from build123d import *

# Parameters (mm, degrees)
SKETCH1_W           = 40
SKETCH1_H           = 28
BOSS_EXTRUDE1_DEPTH = 10
SKETCH2_W           = 40
SKETCH2_H           = 1.6
CUT_EXTRUDE1_DEPTH  = 5
SKETCH3_W           = 24
SKETCH3_H           = 10
CUT_EXTRUDE2_DEPTH  = 27.381811917
SKETCH4_W           = 4
SKETCH4_H           = 26.4
CUT_EXTRUDE3_DEPTH  = 5
FILLET1_R           = 2
FILLET2_R           = 1
CHAMFER2_SIZE       = 0.6


with BuildPart() as part:
    # Sketch1 → Boss-Extrude1 (new body)
    with BuildSketch(Plane(origin=(0, 0, 0), x_dir=(1, 0, 0), z_dir=(0, 1, 0))):
        Rectangle(SKETCH1_W, SKETCH1_H)
    extrude(amount=BOSS_EXTRUDE1_DEPTH)

    # Sketch2 → Cut-Extrude1 (cut)
    with BuildSketch(Plane.XZ):
        with Locations((0, 13.2)):
            Rectangle(SKETCH2_W, SKETCH2_H)
    extrude(amount=-CUT_EXTRUDE1_DEPTH, mode=Mode.SUBTRACT)

    # Sketch3 → Cut-Extrude2 (cut, through all)
    with BuildSketch(Plane(origin=(0, 10, 0), x_dir=(1, 0, 0), z_dir=(0, 1, 0))):
        with Locations((0, -14)):
            Rectangle(SKETCH3_W, SKETCH3_H)
    extrude(amount=-CUT_EXTRUDE2_DEPTH, mode=Mode.SUBTRACT)

    # Sketch4 → Cut-Extrude3 (cut)
    with BuildSketch(Plane.XZ):
        with Locations((-18, -0.8)):
            Rectangle(SKETCH4_W, SKETCH4_H)
        with Locations((18, -0.8)):
            Rectangle(SKETCH4_W, SKETCH4_H)
    extrude(amount=-CUT_EXTRUDE3_DEPTH, mode=Mode.SUBTRACT)

    # Fillet1
    fillet1_edges = [part.edges().sort_by_distance(p)[0] for p in [
        (12, 5, 9),
        (-12, 5, 9),
    ]]
    fillet(fillet1_edges, radius=FILLET1_R)

    # Fillet2
    fillet2_edges = [part.edges().sort_by_distance(p)[0] for p in [
        (12, 7.5, 14),
        (12, 2.5, 12.4),
        (-12, 7.5, 14),
        (-12, 2.5, 12.4),
        (-16, 2.5, 12.4),
        (-16, 2.5, -14),
        (16, 2.5, -14),
        (16, 2.5, 12.4),
        (20, 7.5, 14),
        (-20, 7.5, 14),
        (-20, 7.5, -14),
        (20, 7.5, -14),
    ]]
    fillet(fillet2_edges, radius=FILLET2_R)

    # Chamfer2
    chamfer2_edges = [part.edges().sort_by_distance(p)[0] for p in [
        (0, 0, -14),
        (0, 10, -14),
        (17, 5, -14),
        (-12, 10, 12),
        (12, 10, 12),
        (16, 10, 14),
        (20, 10, 0),
        (-16, 10, 14),
        (-12.292893219, 10, 13.707106781),
        (-19.707106781, 10, 13.707106781),
        (12.292893219, 10, 13.707106781),
        (19.707106781, 10, 13.707106781),
        (19.707106781, 10, -13.707106781),
        (-19.707106781, 10, -13.707106781),
        (-16, 0, -0.8),
        (16, 0, -0.8),
        (14, 0, 12.4),
        (12, 0, 11.2),
        (-12, 0, 11.2),
        (-14, 0, 12.4),
        (-12.292893219, 0, 12.107106781),
        (-15.707106781, 0, 12.107106781),
        (12.292893219, 0, 12.107106781),
        (15.707106781, 0, 12.107106781),
        (15.707106781, 0, -13.707106781),
        (-15.707106781, 0, -13.707106781),
        (20, 5, 0),
        (16, 5, 14),
        (12.292893219, 5, 13.707106781),
        (19.707106781, 5, 13.707106781),
        (19.707106781, 5, -13.707106781),
        (12, 5, 12.2),
        (-12, 5, 12.2),
        (-17, 5, -14),
        (0, 10, 9),
        (0, 0, 9),
        (11.414213562, 10, 9.585786438),
        (11.414213562, 0, 9.585786438),
        (-11.414213562, 10, 9.585786438),
        (-11.414213562, 0, 9.585786438),
        (-20, 5, 0),
        (-20, 10, 0),
        (-16, 5, 14),
        (-12.292893219, 5, 13.707106781),
        (-19.707106781, 5, 13.707106781),
        (-19.707106781, 5, -13.707106781),
    ]]
    chamfer(chamfer2_edges, length=CHAMFER2_SIZE)


solid = part.part
The listing builds one solid part. Answer for the finished solid, in the listing's coordinates (mm). A direction names the side the tool comes from. Coordinates: 2 decimals unless noted, no trailing zeros. Write each loop counter-clockwise with the first axis right and the second up, starting at its lowest first coordinate (ties: lowest second). Pieces come first, ordered by that corner, then holes. Notation, with made-up numbers: M -9.75,78 L 14.25,78 A25 ccw 14.25,110 Z; hole C 4,55 d6. An arc over 180 degrees is marked long. Write each question's results on one line, items separated by ' | '.
Item 1: Consider probe 1 along Y at (x, z) = (-18, -10.25); probe 2 along Z at (x, y) = (8, 9.25); probe 3 along Z at (x, y) = (13, 1). Determine where each line is inside the solid, lowest interval first. Write a range as [from, to].
Answer below:
probe 1: [5, 10] | probe 2: [-14, 9] | probe 3: [-14, 12.4]
Item 2: Given P1, Ø1.3, axis at y = 3, z = 1, coming from the +X side; P2, Ø1, axis at x = 13.5, y = 3.5, coming from the +Z side; P3, Ø1, axis at y = 3.5, z = 11.5, coming from the -X side, each flat-ended and moving along its own axis, determine where each tip first touches the part or whether it passes through.
Answer below:
P1: x = 16 | P2: z = 12.4 | P3: x = -16
Item 3: The part is cut by section D-D on x = 14. Determine the outline of the cut face in (y, z), and give its area (3 significant figures).
Answer below:
outline: M 0,-13.4 L 0.6,-14 L 9.4,-14 L 10,-13.4 L 10,13.4 L 9.4,14 L 5.6,14 L 5,13.4 L 5,12.4 L 0.6,12.4 L 0,11.8 Z | area: 271 mm2
Item 4: The part is cut by section C-C on y = 3.25. Determine the outline of the cut face in (x, z), and give its area (3 significant figures).
Answer below:
outline: M -16,-13 A1 ccw -15,-14 L 15,-14 A1 ccw 16,-13 L 16,11.4 A1 ccw 15,12.4 L 13,12.4 A1 ccw 12,11.4 L 12,11 A2 cw 10,9 L -10,9 A2 cw -12,11 L -12,11.4 A1 ccw -13,12.4 L -15,12.4 A1 ccw -16,11.4 Z | area: 764 mm2
Item 5: The part is cut by section B-B on z = -10.5. Determine the outline of the cut face in (x, y), and give its area (3 significant figures).
Answer below:
outline: M -20,5.6 L -19.4,5 L -16,5 L -16,0.6 L -15.4,0 L 15.4,0 L 16,0.6 L 16,5 L 19.4,5 L 20,5.6 L 20,9.4 L 19.4,10 L -19.4,10 L -20,9.4 Z | area: 359 mm2
Item 6: Which of the six approach directions +Z, -Z, +X, -X, +Y, -Y give full straight-line access (tool end or side, diameter ignored) to faces 1 (the face through (-12.285, 3.065, 12.099)), 2 (the face through (-15.699, 3.135, -13.715)), 3 (the face through (19.699, 7.527, 13.715))?
Answer below:
face 1: +Z, -Y | face 2: -Z, -X, -Y | face 3: +Z, +X, +Y, -Y
Item 7: The part is cut by section A-A on x = 3. Determine the outline of the cut face in (y, z), and give its area (3 significant figures).
Answer below:
outline: M 0,-13.4 L 0.6,-14 L 9.4,-14 L 10,-13.4 L 10,8.4 L 9.4,9 L 0.6,9 L 0,8.4 Z | area: 229 mm2
